Part model, mm, in its own coordinate system. A direction names the side the tool comes from. Round coordinates to 2 decimals unless told otherwise and drop trailing zeros. Loops run counter-clockwise (first coordinate to the right, second up) from the corner with the lowest first, then second, coordinate; pieces in that order, holes last.
from build123d import *

# Parameters (mm, degrees)
CYLINDER017_R     = 1
CYLINDER017_DEPTH = 10
CYLINDER018_R     = 1
CYLINDER018_DEPTH = 10
CYLINDER014_R     = 1.1
CYLINDER014_DEPTH = 12
CYLINDER_R        = 6.3
CYLINDER_DEPTH    = 52
PAD007_DEPTH      = 30
PAD006_DEPTH      = 30
PAD013_DEPTH      = 3
PAD012_DEPTH      = 3


with BuildPart() as cilindro005:
    # Cylinder017 → Cylinder017 (new body)
    with BuildSketch(Plane(origin=(-28, 0, -4), x_dir=(1, 0, 0), z_dir=(0, 0, 1))):
        Circle(CYLINDER017_R)
    extrude(amount=CYLINDER017_DEPTH)


with BuildPart() as fusion001010:
    # Cylinder018 → Cylinder018 (new body)
    with BuildSketch(Plane(origin=(-56, 0, -4), x_dir=(1, 0, 0), z_dir=(0, 0, 1))):
        Circle(CYLINDER018_R)
    extrude(amount=CYLINDER018_DEPTH)

    # Fusion001010: union Cilindro005
    add(cilindro005.part)


with BuildPart() as cilindro:
    # Cylinder014 → Cylinder014 (new body)
    with BuildSketch(Plane.XY):
        Circle(CYLINDER014_R)
    extrude(amount=CYLINDER014_DEPTH)


with BuildPart() as eje:
    # Cylinder → Cylinder (new body)
    with BuildSketch(Plane(origin=(-84, 0, -28), x_dir=(1, 0, 0), z_dir=(0, 0, 1))):
        Circle(CYLINDER_R)
    extrude(amount=CYLINDER_DEPTH)


with BuildPart() as base002:
    # Sketch009 → Pad007 (new body)
    with BuildSketch(Plane.XY):
        with BuildLine():
            Line((0, 18), (-84, 18))
            ThreePointArc((-84, 18), (-102, 0), (-84, -18))
            Line((0, -18), (-84, -18))
            Line((0, 18), (0, -18))
        make_face()
    extrude(amount=PAD007_DEPTH)


with BuildPart() as base002_1:
    # Body011 placement: moved
    add(base002.part.moved(Location((0, 0, 4))))


with BuildPart() as cut013007:
    # Sketch008 → Pad006 (new body)
    with BuildSketch(Plane.XY):
        with BuildLine():
            Line((0, 20), (-84, 20))
            ThreePointArc((-84, 20), (-104, 0), (-84, -20))
            Line((0, -20), (-84, -20))
            Line((0, 20), (0, -20))
        make_face()
    extrude(amount=PAD006_DEPTH)

    # Cut017: cut Base002
    add(base002_1.part, mode=Mode.SUBTRACT)

    # Cut018: cut Eje
    add(eje.part, mode=Mode.SUBTRACT)

    # Fusion001006: union Cilindro
    add(cilindro.part)

    # Cut013007: cut Fusion001010
    add(fusion001010.part, mode=Mode.SUBTRACT)


with BuildPart() as tapa004:
    # Sketch019 → Pad013 (new body)
    with BuildSketch(Plane.XY):
        with BuildLine():
            Line((0, 15.7), (-83.4, 15.7))
            ThreePointArc((-83.4, 15.7), (-99.1, 0), (-83.4, -15.7))
            Line((0, -15.7), (-83.4, -15.7))
            Line((0, 15.7), (0, -15.7))
        make_face()
    extrude(amount=PAD013_DEPTH)


with BuildPart() as tapa004_1:
    # Body016 placement: moved
    add(tapa004.part.moved(Location((0, 0, 26))))


with BuildPart() as fusion001014:
    # Sketch018 → Pad012 (new body)
    with BuildSketch(Plane.XY):
        with BuildLine():
            Line((0, 19), (-83.4, 19))
            ThreePointArc((-83.4, 19), (-102.4, 0), (-83.4, -19))
            Line((0, -19), (-83.4, -19))
            Line((0, 19), (0, -19))
        make_face()
    extrude(amount=PAD012_DEPTH)


with BuildPart() as fusion001014_1:
    # Body015 placement: moved
    add(fusion001014.part.moved(Location((0, 0, 26))))

    # Cut013003: cut Tapa004
    add(tapa004_1.part, mode=Mode.SUBTRACT)


with BuildPart() as fusion001014_2:
    # Cut013003 placement: moved
    add(fusion001014_1.part.moved(Location((0, 0, -3.3))))

    # Fusion001014: union Cut013007
    add(cut013007.part)


with BuildPart() as part_mirroring009:
    # Part__Mirroring009: instance of Fusion001014
    add(fusion001014_2.part.mirror(Plane(origin=(0, 0, 0), x_dir=(0, -1, 0), z_dir=(1, 0, 0))))


solid = part_mirroring009.part
1) Tool access for faces 1 (the face through (41, -18, 13)), 2 (the face through (104, 0, 15)), 3 (the face through (99.096, 0.345, 24.179)), 4 (the face through (0, -18.2, 8.3)), 5 (the face through (-1.05, 0.33, 7.25)): list every direction of +Z, -Z, +X, -X, +Y, -Y with a clear straight run to the whole face (end or side of a thin tool).
Values:
face 1: -X
face 2: +Z, -Z, +X
face 3: +Z, -X
face 4: +Z, -Z, -X, -Y
face 5: +Z
2) Drop flat-ended pins along their axis: pin 1 Ø4 at (y, z) = (1, 17) entering from +X; pin 2 Ø2 at (x, y) = (58, -10.5) entering from +Z; pin 3 Ø1.1 at (x, y) = (0, 0) entering from +Z; pin 4 Ø5 at (x, y) = (21, -13) entering from -Z. Give the stop position or say it passes through.
Values:
pin 1: stops at x = 104
pin 2: stops at z = 4
pin 3: stops at z = 12
pin 4: stops at z = 0
3) Slice it at A-A, the plane x = 28. Give the cut face in (y, z), then the cut area to 3 significant figures.
Values:
outline: (-20, 0) - (-1, 0) - (-1, 4) - (-18, 4) - (-18, 22.7) - (-15.7, 22.7) - (-15.7, 25.7) - (-18, 25.7) - (-18, 30) - (-20, 30) - close; (1, 0) - (20, 0) - (20, 30) - (18, 30) - (18, 25.7) - (15.7, 25.7) - (15.7, 22.7) - (18, 22.7) - (18, 4) - (1, 4) - close
area: 270 mm2
4) Slice it at C-C, the plane y = 3.5. Give the cut face in (x, z).
Values:
outline: (0, 0) - (78.76, 0) - (78.76, 4) - (0, 4) - close; (89.24, 0) - (103.69, 0) - (103.69, 30) - (101.66, 30) - (101.66, 25.7) - (98.7, 25.7) - (98.7, 22.7) - (101.66, 22.7) - (101.66, 4) - (89.24, 4) - close
5) Wall check: line 1 along X through (y, z) = (0, 2.6); line 2 along Y through (x, z) = (55, 21); line 3 along Y through (x, z) = (28, 1.1). Give the ranges that are in metal, low to high.
Values:
line 1: x = -1.1 to 27, 29 to 55, 57 to 77.7, 90.3 to 104
line 2: y = -20 to -18, 18 to 20
line 3: y = -20 to -1, 1 to 20
6) Slice it at B-B, the plane z = 8. Give the cut face in (x, y), then the cut area to 3 significant figures.
Values:
outline: circle Ø2.2 at (0, 0); (0, -20) - (84, -20) arc R20 ccw to (84, 20) - (0, 20) - (0, 18) - (84, 18) arc R18 cw to (84, -18) - (0, -18) - close
area: 459 mm2
7) Mould opens along Z. For faces 6 (the face through (41, 18, 13)), 7 (the face through (52, 0, 0)), 8 (the face through (41, 15.7, 24)) say: released by +Z, released by -Z, zero draft, split by the parting line, or undercut.
Values:
face 6: undercut
face 7: released by -Z
face 8: zero draft
8) Slice it at D-D, the plane z = 2.5. Give the cut face in (x, y).
Values:
outline: (0, -20) - (84, -20) arc R20 ccw to (84, 20) - (0, 20) - (0, 1.1) arc R1.1 ccw to (0, -1.1) - close; hole circle Ø2 at (28, 0); hole circle Ø2 at (56, 0); hole circle Ø12.6 at (84, 0)
